from build123d import *

# Parameters (mm, degrees)
BOSS_EXTRUDE1_DEPTH = 10
CUT_EXTRUDE1_DEPTH  = 7
SKETCH4_R           = 4
CUT_EXTRUDE2_DEPTH  = 5
SKETCH5_R           = 2.5
CUT_EXTRUDE3_DEPTH  = 6
SKETCH6_R           = 2.5
CUT_EXTRUDE4_DEPTH  = 11
SKETCH7_R           = 2.5
CUT_EXTRUDE5_DEPTH  = 11
CHAMFER1_SIZE       = 1
FILLET1_R           = 1


with BuildPart() as part:
    # Sketch2 → Boss-Extrude1 (new body)
    with BuildSketch(Plane(origin=(0, 0, 0), x_dir=(1, 0, 0), z_dir=(0, 1, 0))):
        Polygon((0, 0), (40, 0), (40, 100), (55, 100), (55, 220), (50, 225), (-10, 225), (-15, 220), (-15, 100), (0, 100), align=None)
    extrude(amount=BOSS_EXTRUDE1_DEPTH)

    # Sketch3 → Cut-Extrude1 (cut)
    with BuildSketch(Plane.XZ):
        Polygon((-15, -220), (-10, -225), (50, -225), (55, -220), (55, -170), (-15, -170), align=None)
    extrude(amount=-CUT_EXTRUDE1_DEPTH, mode=Mode.SUBTRACT)

    # Sketch4 → Cut-Extrude2 (cut)
    with BuildSketch(Plane(origin=(0, 10, 0), x_dir=(1, 0, 0), z_dir=(0, 1, 0))):
        with Locations((10, 25)):
            Circle(SKETCH4_R)
        with Locations((30, 25)):
            Circle(SKETCH4_R)
        with Locations((10, 90)):
            Circle(SKETCH4_R)
        with Locations((30, 90)):
            Circle(SKETCH4_R)
    extrude(amount=-CUT_EXTRUDE2_DEPTH, mode=Mode.SUBTRACT)

    # Sketch5 → Cut-Extrude3 (cut, through all)
    with BuildSketch(Plane(origin=(0, 5, 0), x_dir=(1, 0, 0), z_dir=(0, 1, 0))):
        with Locations((30, 90)):
            Circle(SKETCH5_R)
        with Locations((10, 90)):
            Circle(SKETCH5_R)
        with Locations((10, 25)):
            Circle(SKETCH5_R)
        with Locations((30, 25)):
            Circle(SKETCH5_R)
    extrude(amount=-CUT_EXTRUDE3_DEPTH, mode=Mode.SUBTRACT)

    # Sketch6 → Cut-Extrude4 (cut, through all)
    with BuildSketch(Plane(origin=(0, 10, 0), x_dir=(1, 0, 0), z_dir=(0, 1, 0))):
        with Locations((50, 190)):
            Circle(SKETCH6_R)
        with Locations((-10, 190)):
            Circle(SKETCH6_R)
        with Locations((-10, 120)):
            Circle(SKETCH6_R)
        with Locations((50, 120)):
            Circle(SKETCH6_R)
    extrude(amount=-CUT_EXTRUDE4_DEPTH, mode=Mode.SUBTRACT)

    # Sketch7 → Cut-Extrude5 (cut, through all)
    with BuildSketch(Plane(origin=(0, 10, 0), x_dir=(1, 0, 0), z_dir=(0, 1, 0))):
        with Locations((32, 8)):
            Circle(SKETCH7_R)
        with Locations((7.000002149, 8.010365644)):
            Circle(SKETCH7_R)
    extrude(amount=-CUT_EXTRUDE5_DEPTH, mode=Mode.SUBTRACT)

    # Chamfer1
    chamfer1_edges = [part.edges().sort_by_distance(p)[0] for p in [
        (40, 10, -50),
        (0, 10, -50),
        (20, 10, 0),
    ]]
    chamfer(chamfer1_edges, length=CHAMFER1_SIZE)

    # Fillet1
    fillet1_edges = [part.edges().sort_by_distance(p)[0] for p in [
        (55, 10, -160),
        (-15, 10, -160),
    ]]
    fillet(fillet1_edges, radius=FILLET1_R)


solid = part.part
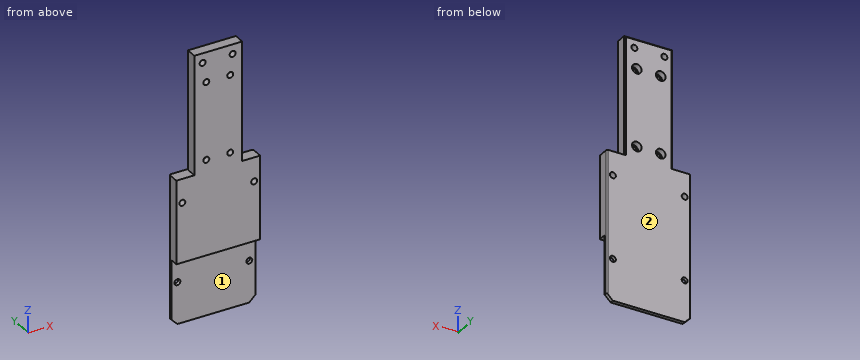
Part model, mm, in its own coordinate system. Face numbers are marked on the shaded views. A direction names the side the tool comes from. Give positions to 0.01 mm unless a question says otherwise; leave off trailing zeros. Write each loop counter-clockwise with the first axis right and the second up, starting at its lowest first coordinate (ties: lowest second). Pieces come first, ordered by that corner, then holes.
1) Cut at A-A on z = -190. Write the cut outline in (x, y).
Resolved:
outline: (-15, 7) - (-12.5, 7) - (-12.5, 10) - (-14, 10) arc R1 ccw to (-15, 9) - close; (-7.5, 7) - (47.5, 7) - (47.5, 10) - (-7.5, 10) - close; (52.5, 7) - (55, 7) - (55, 9) arc R1 ccw to (54, 10) - (52.5, 10) - close
2) Cut at B-B on x = 36.5. Write the cut outline in (y, z), then the cut area to 3 significant figures.
Resolved:
outline: (0, -170) - (7, -170) - (7, -225) - (10, -225) - (10, -1) - (9, 0) - (0, 0) - close
area: 1,860 mm2
3) Cut at D-D on z = -19. Write the cut outline in (x, y), then the cut area to 3 significant figures.
Resolved:
outline: (0, 0) - (40, 0) - (40, 9) - (39, 10) - (1, 10) - (0, 9) - close
area: 399 mm2
4) Pin check, flat tips, straight feed: pin 1 (3 mm diameter, centred on x = 43.5, y = 5.5, fed in from +Z); pin 2 (6.5 mm diameter, centred on x = 30, z = -90, fed in from +Y); pin 3 (5 mm diameter, centred on x = 26, z = -62.5, fed in from -Y); pin 4 (3 mm diameter, centred on x = 23, y = 3, fed in from -Z). Stop position of each tip, or through.
Resolved:
pin 1: stops at z = -100
pin 2: stops at y = 5
pin 3: stops at y = 0
pin 4: stops at z = -170
5) Which spindle directions (+Z, -Z, +X, -X, +Y, -Y) get a long thin tool onto all of the face, cutting with end or side? Do the marked faces 1 and 2. Say none if no direction does.
Resolved:
face 1: -Z, +X, -X, -Y
face 2: +Z, -Z, +X, -X, +Y
6) Probe L1, parallel to Z at x = -10, y = 8.35; L2, parallel to X at y = 7, z = -90; L3, parallel to Z at x = 8.5, y = 6.5. List the from-to ranges inside material, lowest first.
Resolved:
L1: z = -225 to -192.5, -187.5 to -122.5, -117.5 to -100
L2: x = 0 to 6, 14 to 26, 34 to 40
L3: z = -170 to -93.71, -86.29 to -28.71, -21.29 to -10.01, -6.01 to 0
7) Cut at C-C on y = 3.25. State how many separate pieces and enclosed holes the cut face has, then the cut area to 3 significant figures.
Resolved:
separate pieces: 1
enclosed holes: 8
area: 8,740 mm2
